Verification items for the finished model (mm, model axes). A direction names the side the tool comes from. Round coordinates to 2 decimals unless told otherwise and drop trailing zeros. Write each loop counter-clockwise with the first axis right and the second up, starting at its lowest first coordinate (ties: lowest second). Pieces come first, ordered by that corner, then holes. Notation, with made-up numbers: M -14,-37.75 L 32,-37.75 A26 ccw 32,-4.75 Z; hole C -15,-31.75 d1. An arc over 180 degrees is marked long. Use a Markdown table: item, result. Add a question column.
Autodesk Inventor part; units mm, degrees
ref_plane "YZ Plane" through (0, 0, 0) normal (1, 0, 0) x (0, 1, 0)
ref_plane "XZ Plane" through (0, 0, 0) normal (0, 1, 0) x (-1, 0, 0)
ref_plane "XY Plane" through (0, 0, 0) normal (0, 0, 1) x (1, 0, 0)
sketch "Sketch1" plane through (0, 0, 0) normal (0, 0, 1) x (1, 0, 0)
  line L0 (0, 0) -> (30, 0)
  line L1 (30, 0) -> (30, 42.4)
  line L2 (30, 42.4) -> (0, 42.4)
  line L3 (0, 42.4) -> (0, 0)
  circle A0 centre (15, 21.2) radius 7.5
  dimension "d0" = 42.4
  dimension "d1" = 30
  dimension "d2" = 15
  dimension "d3" = 21.2
  dimension "d4" = 15
extrude "Extrusion1" add sketch "Sketch1" along normal blind 20
sketch "Sketch2" plane through (0, 0, 0) normal (-1, 0, 0) x (0, 0, 1)
  line L0 (20, 0) -> (20, 42.4)
  line L1 (0, 42.4) -> (20, 42.4)
  line L2 (0, 42.4) -> (0, 0)
  line L3 (0, 0) -> (20, 0)
  circle A0 centre (4, 33.4) radius 2.05
  circle A1 centre (16, 33.4) radius 2.05
  circle A2 centre (4, 9) radius 2.05
  circle A3 centre (16, 9) radius 2.05
  dimension "d7" = 4.1
  dimension "d8" = 4
  dimension "d9" = 4
  dimension "d10" = 4
  dimension "d11" = 4
  dimension "d12" = 9
  dimension "d13" = 9
  dimension "d14" = 9
  dimension "d15" = 9
extrude "Extrusion6" cut sketch "Sketch2" against normal through all contours A0 | A1 | A2 | A3
fillet "Fillet3" radius 3 3 edges at (0, 21.2, 20) (0, 21.2, 0) (0, 0, 10)
fillet "Fillet4" radius 3 4 edges at (0.8787, 0.8787, 19.1213) (16.5, 0, 20) (0.8787, 0.8787, 0.8787) (16.5, 0, 0)
sketch "Sketch6" plane through (0, 0, 20) normal (0, 0, 1) x (1, 0, 0)
  circle A0 centre (15, 21.2) radius 7.5
  line L0 (30, 42.4) -> (30, 3)
  line L1 (0, 24) -> (0, 19.2632)
  line L2 (30, 24) -> (25.7429, 24)
  line L3 (4.2571, 24) -> (0, 24)
  arc A1 (25.7429, 24) -> (4.2571, 24) centre (15, 21.2) ccw
  line L4 (0, 19.2632) -> (7.7544, 19.2632)
  line L5 (22.2456, 19.2632) -> (30, 19.2632)
  point P0 (0, 0)
extrude "Extrusion7" cut sketch "Sketch6" against normal blind 4 contours A0 L4 L1 L3 A1 L2 L0 L5
sketch "Sketch3" plane through (0, 0, 0) normal (0, -1, 0) x (1, 0, 0)
  line L0 (30, 20) -> (0, 20)
  line L1 (0, 0) -> (0, 20)
  line L2 (30, 0) -> (30, 20)
  circle A0 centre (5, 10) radius 2.05
  circle A1 centre (25, 10) radius 2.05
  dimension "d18" = 4.1
  dimension "d19" = 5
  dimension "d20" = 5
  dimension "d21" = 10
  dimension "d22" = 10
sketch "Sketch4" plane through (0, 0, 0) normal (-1, 0, 0) x (0, 0, 1)
  circle A0 centre (16, 9) radius 2.05
  circle A1 centre (4, 9) radius 2.05
  circle A2 centre (16, 33.4) radius 2.05
  circle A3 centre (4, 33.4) radius 2.05
  circle A4 centre (4, 33.4) radius 3.75
  circle A5 centre (16, 33.4) radius 3.75
  circle A6 centre (4, 9) radius 3.75
  circle A7 centre (16, 9) radius 3.75
  dimension "d25" = 7.5
sketch "Sketch5" plane through (0, 0, 0) normal (0, -1, 0) x (1, 0, 0)
  circle A0 centre (25, 10) radius 2.05
  circle A1 centre (5, 10) radius 2.05
  circle A2 centre (5, 10) radius 3.75
  circle A3 centre (25, 10) radius 3.75
  dimension "d28" = 7.5
equation "\"d3\" = 0.5 * d0"
equation "\"d9\" = d8"
equation "\"d10\" = d8"
equation "\"d11\" = d8"
equation "\"d13\" = d12"
equation "\"d14\" = d12"
equation "\"d15\" = d12"
equation "\"d20\" = d19"
properties part number "V5 multi bottom"
1. Depth check by flat-ended pin: pin 1 Ø1 at (x, z) = (20.5, 11.5) entering from -Y; pin 2 Ø2.5 at (y, z) = (9, 4) entering from -X; pin 3 Ø1.5 at (y, z) = (25.5, 18) entering from -X; pin 4 Ø6 at (x, y) = (11, 25.5) entering from +Z. Enter the tip coordinate at first touch or a pass-through.
2. Cross-section at D-D on x = 27. Enter the section's corners in (y, z), plus the area to 3 significant figures.
3. Cross-section at C-C on y = 26.5. Enter the section's corners in (x, z) (3 decimals), plus the area to 3 significant figures.
4. Cross-section at A-A on z = 4. Enter the section's corners in (x, y), plus the area to 3 significant figures.
5. Release check for a two-part mould opening along X. For faces 1 (the flat face through (0, 23, 10)), 2 (the cylindrical face through (15.2, 32.3, 18)), 3 (the cylindrical face through (14.8, 34.8, 14.5)) record: +X half, -X half, draft (parallel to the pull), parting line (faces both ways), or undercut.
6. Scan lines: line 1 along Z through (x, y) = (9.5, 33.5); line 2 along Y through (x, z) = (21, 17); line 3 along X through (y, z) = (21.2, 8.5). Record each from-to range of solid material in increasing order. Write a range as from..to.
7. Cross-section at B-B on x = 12.5. Enter the section's corners in (y, z), plus the area to 3 significant figures.
8. Access from +Z, -Z, +X, -X, +Y, -Y to the whole of each face (thin tool, end or side, straight path). Record for faces 4 (the flat face through (4, 19.263, 18)), 5 (the flat face through (15, 29, 16)), 6 (the cylindrical face through (0.9, 0.86, 9.9)).
Answer:
| question | item | result |
|---|---|---|
| 1 | pin 1 | stops at y = 0 |
| 1 | pin 2 | passes through |
| 1 | pin 3 | stops at x = 0.01 |
| 1 | pin 4 | stops at z = 16 |
| 2 | outline | M 0,3 A3 ccw 3,0 L 42.4,0 L 42.4,20 L 24,20 L 24,16 L 19.26,16 L 19.26,20 L 3,20 A3 ccw 0,17 Z; hole C 9,4 d4.1; hole C 9,16 d4.1; hole C 33.4,4 d4.1; hole C 33.4,16 d4.1 |
| 2 | area | 772 mm^2 |
| 3 | outline | M 0,3 A3 ccw 3,0 L 9.693,0 L 9.693,16 L 5.245,16 L 5.245,20 L 3,20 A3 ccw 0,17 Z; M 20.307,0 L 30,0 L 30,20 L 24.755,20 L 24.755,16 L 20.307,16 Z |
| 3 | area | 348 mm^2 |
| 4 | outline | M 0,3 A3 ccw 3,0 L 30,0 L 30,6.95 L 0,6.95 Z; M 0,11.05 L 30,11.05 L 30,31.35 L 0,31.35 Z; M 0,35.45 L 30,35.45 L 30,42.4 L 0,42.4 Z; hole C 15,21.2 d15 |
| 4 | area | 847 mm^2 |
| 5 | face 1 | -X half |
| 5 | face 2 | undercut |
| 5 | face 3 | draft |
| 6 | line 1 | z = 0..1.95, 6.05..13.95, 18.05..20 |
| 6 | line 2 | y = 0..7.21, 10.79..16.7, 30.54..31.61, 35.19..42.4 |
| 6 | line 3 | x = 0..7.5, 22.5..30 |
| 7 | outline | M 0,3 A3 ccw 3,0 L 14.13,0 L 14.13,20 L 3,20 A3 ccw 0,17 Z; M 28.27,0 L 42.4,0 L 42.4,20 L 32.02,20 L 32.02,17.51 A2.05 cw long 31.35,16 L 28.27,16 Z; hole C 9,4 d4.1; hole C 9,16 d4.1; hole C 33.4,4 d4.1 |
| 7 | area | 494 mm^2 |
| 8 | face 4 | +Z, +X, -X |
| 8 | face 5 | +Z |
| 8 | face 6 | +Z, -Z, -X, -Y |
